from build123d import *

# Parameters (mm, degrees)
SKETCH1_W                        = 615.95
SKETCH1_H                        = 279.4
BOSS_EXTRUDE1_DEPTH              = 3.175
SKETCH2_W                        = 641.35
SKETCH2_H                        = 47.625
BOSS_EXTRUDE2_DEPTH              = 3.175
FILLET1_R                        = 3.175
CUT_EXTRUDE1_DEPTH               = 4.175
F_17_64_0_26563_DIAMETER_HOLE1_D = 6.747002


with BuildPart() as part:
    # Sketch1 → Boss-Extrude1 (new body)
    with BuildSketch(Plane(origin=(0, 0, 0), x_dir=(1, 0, 0), z_dir=(0, 1, 0))):
        with Locations((307.975, -139.7)):
            Rectangle(SKETCH1_W, SKETCH1_H)
    extrude(amount=BOSS_EXTRUDE1_DEPTH)

    # Sketch2 → Boss-Extrude2 (add, through all)
    with BuildSketch(Plane(origin=(0, 3.175, 0), x_dir=(1, 0, 0), z_dir=(0, 1, 0))):
        with Locations((307.975, -88.9)):
            Rectangle(SKETCH2_W, SKETCH2_H)
        with Locations((307.975, -190.5)):
            Rectangle(SKETCH2_W, SKETCH2_H)
    extrude(amount=-BOSS_EXTRUDE2_DEPTH)

    # Fillet1
    fillet1_edges = [part.edges().sort_by_distance(p)[0] for p in [
        (628.65, 1.5875, 112.7125),
        (-12.7, 1.5875, 65.0875),
        (628.65, 1.5875, 65.0875),
        (0, 1.5875, 112.7125),
        (615.95, 1.5875, 112.7125),
        (-12.7, 1.5875, 112.7125),
        (0, 1.5875, 65.0875),
        (615.95, 1.5875, 65.0875),
        (628.65, 1.5875, 214.3125),
        (-12.7, 1.5875, 166.6875),
        (628.65, 1.5875, 166.6875),
        (0, 1.5875, 214.3125),
        (615.95, 1.5875, 214.3125),
        (-12.7, 1.5875, 214.3125),
        (0, 1.5875, 166.6875),
        (615.95, 1.5875, 166.6875),
    ]]
    fillet(fillet1_edges, radius=FILLET1_R)

    # Sketch3 → Cut-Extrude1 (cut, through all)
    with BuildSketch(Plane(origin=(0, 3.175, 0), x_dir=(1, 0, 0), z_dir=(0, 1, 0))):
        with BuildLine():
            Line((202.8825, -192.0875), (202.8825, -87.3125))
            ThreePointArc((202.8825, -87.3125), (204.7875, -85.4075), (206.6925, -87.3125))
            Line((206.6925, -87.3125), (206.6925, -192.0875))
            ThreePointArc((206.6925, -192.0875), (204.7875, -193.9925), (202.8825, -192.0875))
        make_face()
        with BuildLine():
            Line((409.2575, -192.0875), (409.2575, -87.3125))
            ThreePointArc((409.2575, -87.3125), (411.1625, -85.4075), (413.0675, -87.3125))
            Line((413.0675, -87.3125), (413.0675, -192.0875))
            ThreePointArc((413.0675, -192.0875), (411.1625, -193.9925), (409.2575, -192.0875))
        make_face()
    extrude(amount=-CUT_EXTRUDE1_DEPTH, mode=Mode.SUBTRACT)

    # 17/64 (0.26563) Diameter Hole1 (through all)
    with Locations(Plane(origin=(0, 3.175, 0), x_dir=(1, 0, 0), z_dir=(0, 1, 0))):
        with Locations((387.35, -25.4), (228.6, -25.4)):
            Hole(F_17_64_0_26563_DIAMETER_HOLE1_D / 2)


solid = part.part
Read the model definition and answer for the solid it produces. Units are mm, in the model's axes. Give positions to 0.01 mm unless a question says otherwise; leave off trailing zeros. Write each loop counter-clockwise with the first axis right and the second up, starting at its lowest first coordinate (ties: lowest second). Pieces come first, ordered by that corner, then holes. Notation, with made-up numbers: (-20, -30.75) - (34, -30.75) arc R12 ccw to (34, -23.75) - close; hole circle Ø2 at (81.5, -30). An arc over 180 degrees is marked (long way). Use CSV: the item, a comma, the result in double quotes. Start each with the question number.
Item 1: Flat-ended cylindrical pins translate along their axes: P1, Ø1, axis at x = 620.5, y = 2.5, coming from the +Z side; P2, Ø9, axis at x = 387.35, z = 25.4, coming from the +Y side (3 decimals); P3, Ø1, axis at x = -7, y = 2, coming from the -Z side; P4, Ø1, axis at y = 2, z = 127, coming from the +X side. Find the tip coordinate at first contact, or state that the pin passes through.
Item 2: The part is cut by section A-A, the plane z = 137. Count the separate pieces of the cut face and the enclosed holes in it, and give its area (3 significant figures).
Item 3: The part is cut by section C-C, the plane z = 43.5. Give the vertices of the cut face in (x, y) (3 decimals).
Item 4: Consider line 1 (X direction, y = 1.3, z = 25.4); line 2 (X direction, y = 2.85, z = 109); line 3 (Z direction, x = 228.6, y = 1.75). Determine where each line is inside the solid, lowest interval first.
Taken from the geometry:
1,P1,"z = 214.31"
1,P2,"y = 3.175"
1,P3,"z = 65.09"
1,P4,"x = 615.95"
2,separate pieces,"3"
2,enclosed holes,"0"
2,area,"1,930 mm2"
3,outline,"(0, 0) - (615.95, 0) - (615.95, 3.175) - (0, 3.175) - close"
4,line 1,"0 to 225.23, 231.97 to 383.98, 390.72 to 615.95"
4,line 2,"-12.7 to 202.88, 206.69 to 409.26, 413.07 to 628.65"
4,line 3,"0 to 22.03, 28.77 to 279.4"
